Geometry: final body of the model. Coordinates: model frame, mm. Face numbers are marked on the shaded views. A direction names the side the tool comes from. Give positions to 0.01 mm unless a question says otherwise; leave off trailing zeros. Write each loop counter-clockwise with the first axis right and the second up, starting at its lowest first coordinate (ties: lowest second). Pieces come first, ordered by that corner, then holes. Notation, with made-up numbers: (2, -4.75) -> (11, -4.75) arc R21 cw to (11, 27.25) -> close; hole circle Ø6 at (34.25, 31.5). An arc over 180 degrees is marked (long way). Answer as a JSON object with one key per item and string values.
from build123d import *

# Parameters (mm, degrees)
BOSS_EXTRUDE1_DEPTH              = 25
SKETCH4_W                        = 29.345301095
SKETCH4_H                        = 9.5
SKETCH4_W_2                      = 30
BOSS_EXTRUDE2_DEPTH              = 39
SKETCH2_R                        = 4
ACTUATOR_SHAFT_PASSTHROUGH_DEPTH = 54.5
SKETCH7_W                        = 25
SKETCH7_H                        = 27
BOSS_EXTRUDE4_DEPTH              = 60


with BuildPart() as part:
    # Sketch1 → Boss-Extrude1 (new body)
    with BuildSketch(Plane.XY):
        Polygon((-54, 27), (54, 27), (54, -2.5), (24.654698905, -2.5), (24.654698905, -17.5), (54, -17.5), (54, -27), (-54, -27), (-54, 2.5), (-24, 2.5), (-24, 17.5), (-54, 17.5), align=None)
    extrude(amount=BOSS_EXTRUDE1_DEPTH)

    # Sketch4 → Boss-Extrude2 (add)
    with BuildSketch(Plane(origin=(0, 0, 0), x_dir=(-1, 0, 0), z_dir=(0, 0, -1))):
        with Locations((-39.327349453, 2.25)):
            Rectangle(SKETCH4_W, SKETCH4_H)
        with Locations((-39.327349453, -22.25)):
            Rectangle(SKETCH4_W, SKETCH4_H)
        with Locations((39, -2.25)):
            Rectangle(SKETCH4_W_2, SKETCH4_H)
        with Locations((39, 22.25)):
            Rectangle(SKETCH4_W_2, SKETCH4_H)
    extrude(amount=BOSS_EXTRUDE2_DEPTH)

    # Sketch2 → Actuator Shaft Passthrough (cut)
    with BuildSketch(Plane(origin=(0, 27, 0), x_dir=(1, 0, 0), z_dir=(0, 1, 0))):
        with Locations((39.327349452, 24)):
            Circle(SKETCH2_R)
        with Locations((-39, 24)):
            Circle(SKETCH2_R)
    extrude(amount=-ACTUATOR_SHAFT_PASSTHROUGH_DEPTH, mode=Mode.SUBTRACT)

    # Sketch7 → Boss-Extrude4 (add)
    with BuildSketch(Plane.ZY.offset(54)):
        with Locations((12.5, -13.5)):
            Rectangle(SKETCH7_W, SKETCH7_H)
    extrude(amount=BOSS_EXTRUDE4_DEPTH)


solid = part.part
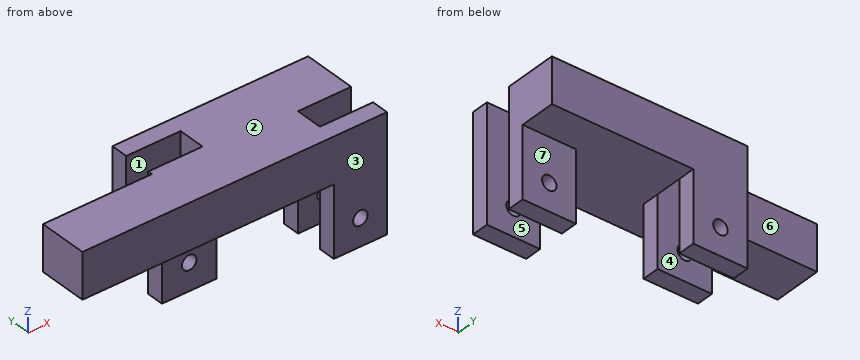
Q1. First-contact query: P1, Ø6.5, axis at x = -39, z = -24, coming from the -Y side; P2, Ø10, axis at y = 9, z = -28, coming from the -X side; P3, Ø16.5, axis at y = 13.5, z = 16, coming from the -X side; P4, Ø10.5, axis at y = 21.5, z = -14.5, coming from the +X side. Flat tips, straight axial feed; report the tip coordinate or a pass-through.
Values:
{"P1": "through", "P2": "x = 24.65", "P3": "x = -54", "P4": "x = -24"}
Q2. Mould query, pull axis Y, two halves, no side actions, for the marked faces 1, 2 and 3. Classes: pulls with the +Y half, pulls with the -Y half, needs draft (parallel to the pull), parting line crosses it, or undercut.
Values:
{"face 1": "undercut", "face 2": "needs draft", "face 3": "pulls with the -Y half"}
Q3. Material intervals for L1, parallel to Z at x = -39, y = -3; L2, parallel to X at y = 0, z = -15; L3, parallel to Y at x = -46, z = -29.5, sorted ascending. Write a range as from..to.
Values:
{"L1": "-39..-28, -20..25", "L2": "-54..-24, 24.65..54", "L3": "-7..2.5, 17.5..27"}
Q4. Cut plane C-C (y = -20). Return the cut outline in (x, z), and give its area (3 significant figures).
Values:
{"outline": "(-114, 0) -> (24.65, 0) -> (24.65, -39) -> (54, -39) -> (54, 25) -> (-114, 25) -> close; hole circle Ø8 at (39.33, -24)", "area": "5,290 mm²"}
Q5. Cut plane B-B (z = -12.5). Return the cut outline in (x, y).
Values:
{"outline": "(-54, -7) -> (-24, -7) -> (-24, 2.5) -> (-54, 2.5) -> close; (-54, 17.5) -> (-24, 17.5) -> (-24, 27) -> (-54, 27) -> close; (24.65, -27) -> (54, -27) -> (54, -17.5) -> (24.65, -17.5) -> close; (24.65, -2.5) -> (54, -2.5) -> (54, 7) -> (24.65, 7) -> close"}
Q6. Set-up query: the marked faces 4, 5, 6 and 7. Return all of +Z, -Z, +X, -X, +Y, -Y with unobstructed straight access to the full face (end or side cutting, diameter ignored); none if empty.
Values:
{"face 4": "+Z, -Z, -X", "face 5": "+Z, -Z, +X", "face 6": "+Z, -Z, -X, +Y", "face 7": "-Z, +X, -X, +Y"}
Q7. Cut plane A-A (x = -39). Return the cut outline in (y, z).
Values:
{"outline": "(-27, 0) -> (-7, 0) -> (-7, -20) -> (2.5, -20) -> (2.5, 25) -> (-27, 25) -> close; (-7, -39) -> (2.5, -39) -> (2.5, -28) -> (-7, -28) -> close; (17.5, -39) -> (27, -39) -> (27, -28) -> (17.5, -28) -> close; (17.5, -20) -> (27, -20) -> (27, 25) -> (17.5, 25) -> close"}
Q8. Cut plane D-D (z = -24). State how many separate pieces and enclosed holes the cut face has, and give its area (3 significant figures).
Values:
{"separate pieces": "8", "enclosed holes": "0", "area": "824 mm²"}
